The model under review builds one solid part; all positions refer to its coordinate system, in mm. A direction names the side the tool comes from. Coordinates: 2 decimals unless noted, no trailing zeros. Order: outer loops, then holes, each group sorted by start corner. A loop starts at its lowest first (then second) coordinate and runs counter-clockwise, first axis right, second up. Notation, with made-up numbers: (54, -28.75) -> (110, -28.75) arc R4 cw to (110, -21.75) -> close; hole circle Ø2 at (26.5, -18.5). An arc over 180 degrees is marked (long way). Use one line per item in the form item = value. Start each with the question number.
(1) For faces 1 (the flat face through (18.5, -17, -56)), 2 (the flat face through (1, -15.5, -37)), 3 (the flat face through (10, -22, -58)), list the 3-axis set-ups (+Z, -Z, +X, -X, +Y, -Y) from which the entire face can be reached by the end or side of a thin tool; tool diameter is ignored.
(2) Take a section at D-D (z = -17). State the section outline as (x, y) points.
(3) Take a section at C-C (y = 1.5). State the section outline as (x, z) points, then the cut area to 3 significant figures.
(4) Wall thickness on line 1 along Y through (x, z) = (25, 1); line 2 along Y through (x, z) = (-10, 2); line 3 along X through (y, z) = (1, 1): over which ranges is each line inside the solid? List them lowest first.
(5) Insertion check: pin 1 Ø7 at (x, y) = (-10, 8) entering from -Z; pin 2 Ø5 at (x, z) = (-12.5, -7) entering from -Y; pin 3 Ø1.6 at (x, z) = (1.5, -50.5) entering from -Y; pin 4 Ø8 at (x, y) = (-10, -12) entering from -Z. Each pin has a flat end and moves straight along its axis. Give the tip position at first contact, or say it passes through.
(6) Mouldability with a two-part tool opening along X and no side actions: class faces 4 (the flat face through (40, -16, -23)), 5 (the flat face through (1, -34, -50)), 6 (the flat face through (-12, -25, -59)), 7 (the cylindrical face through (20, -17, -60.5)) as +X half, -X half, draft (parallel to the pull), parting line (faces both ways), or undercut.
(7) Take a section at B-B (x = 20). State the section outline as (y, z) points, then the cut area to 3 significant figures.
(8) Take a section at A-A (z = -7). State the section outline as (x, y) points, then the cut area to 3 significant figures.
```python
from build123d import *

# Parameters (mm, degrees)
SZKIC2_W                    = 80
SZKIC2_H                    = 37
SZKIC2_R                    = 3
SZKIC2_R_2                  = 2.5
DODANIE_WYCI_GNI_CIE1_DEPTH = 3
ZAOKR_GLENIE1_R             = 5
SZKIC3_W                    = 80
SZKIC3_H                    = 3
DODANIE_WYCI_GNI_CIE2_DEPTH = 75
WYTNIJ_WYCI_GNI_CIE1_REACH  = 94.704
DODANIE_WYCI_GNI_CIE3_DEPTH = 24
SKORUPA8_START              = -10
SKORUPA8_DEPTH              = 20
SZKIC10_W                   = 20
SZKIC10_H                   = 20
WYTNIJ_WYCI_GNI_CIE5_DEPTH  = 3
SZKIC4_5_R                  = 1.5
WYTNIJ_WYCI_GNI_CIE7_DEPTH  = 3
ZAOKR_GLENIE2_R             = 10
WYTNIJ_WYCI_GNI_CIE8_REACH  = 94.704
SZKIC11_R                   = 2.5


# Read off the part's stored shape, not the designer's step: Skorupa8
with BuildPart() as part:
    # Szkic2 → Dodanie-wyciągnięcie1 (new body)
    with BuildSketch(Plane.XY):
        Rectangle(SZKIC2_W, SZKIC2_H)
        with Locations((-10, -12)):
            Circle(SZKIC2_R, mode=Mode.SUBTRACT)
        with Locations((-25, -8.5)):
            Circle(SZKIC2_R_2, mode=Mode.SUBTRACT)
        with Locations((-25, 1.5)):
            Circle(SZKIC2_R_2, mode=Mode.SUBTRACT)
        with Locations((-25, 11.5)):
            Circle(SZKIC2_R_2, mode=Mode.SUBTRACT)
        with Locations(Location((10, -12, 0), (0, 0, 180))):
            Circle(SZKIC2_R, mode=Mode.SUBTRACT)
        with Locations(Location((25, -8.5, 0), (0, 0, 180))):
            Circle(SZKIC2_R_2, mode=Mode.SUBTRACT)
        with Locations(Location((25, 1.5, 0), (0, 0, 180))):
            Circle(SZKIC2_R_2, mode=Mode.SUBTRACT)
        with Locations(Location((25, 11.5, 0), (0, 0, 180))):
            Circle(SZKIC2_R_2, mode=Mode.SUBTRACT)
        with Locations((-10, 8)):
            Circle(SZKIC2_R, mode=Mode.SUBTRACT)
        with Locations(Location((10, 8, 0), (0, 0, 180))):
            Circle(SZKIC2_R, mode=Mode.SUBTRACT)
    extrude(amount=DODANIE_WYCI_GNI_CIE1_DEPTH)

    # Zaokrąglenie1
    zaokr_glenie1_edges = [part.edges().sort_by_distance(p)[0] for p in [
        (-40, 18.5, 1.5),
        (40, 18.5, 1.5),
    ]]
    fillet(zaokr_glenie1_edges, radius=ZAOKR_GLENIE1_R)

    # Szkic3 → Dodanie-wyciągnięcie2 (add)
    with BuildSketch(Plane(origin=(0, 0, 0), x_dir=(-1, 0, 0), z_dir=(0, 0, -1))):
        with Locations((0, -17)):
            Rectangle(SZKIC3_W, SZKIC3_H)
    extrude(amount=DODANIE_WYCI_GNI_CIE2_DEPTH)

    # Szkic4 → Wytnij-wyciągnięcie1 (cut, up to next)
    with BuildSketch(Plane.XZ.offset(18.5), mode=Mode.PRIVATE) as wytnij_wyci_gni_cie1_sk1:
        with BuildLine():
            Line((-21.5, -65), (-21.5, -70))
            ThreePointArc((-21.5, -70), (-20, -71.5), (-18.5, -70))
            Line((-18.5, -70), (-18.5, -65))
            ThreePointArc((-18.5, -65), (-20, -63.5), (-21.5, -65))
        make_face()
    wytnij_wyci_gni_cie1_tool1 = extrude(wytnij_wyci_gni_cie1_sk1.sketch, amount=-WYTNIJ_WYCI_GNI_CIE1_REACH, mode=Mode.PRIVATE) & part.part
    # Szkic4 → Wytnij-wyciągnięcie1 (cut, up to next)
    with BuildSketch(Plane.XZ.offset(18.5), mode=Mode.PRIVATE) as wytnij_wyci_gni_cie1_sk2:
        with BuildLine():
            ThreePointArc((-18.5, -54), (-20, -52.5), (-21.5, -54))
            Line((-21.5, -54), (-21.5, -59))
            ThreePointArc((-21.5, -59), (-20, -60.5), (-18.5, -59))
            Line((-18.5, -59), (-18.5, -54))
        make_face()
    wytnij_wyci_gni_cie1_tool2 = extrude(wytnij_wyci_gni_cie1_sk2.sketch, amount=-WYTNIJ_WYCI_GNI_CIE1_REACH, mode=Mode.PRIVATE) & part.part
    # Szkic4 → Wytnij-wyciągnięcie1 (cut, up to next)
    with BuildSketch(Plane.XZ.offset(18.5), mode=Mode.PRIVATE) as wytnij_wyci_gni_cie1_sk3:
        with BuildLine():
            ThreePointArc((21.5, -54), (20, -52.5), (18.5, -54))
            Line((18.5, -54), (18.5, -59))
            ThreePointArc((18.5, -59), (20, -60.5), (21.5, -59))
            Line((21.5, -59), (21.5, -54))
        make_face()
    wytnij_wyci_gni_cie1_tool3 = extrude(wytnij_wyci_gni_cie1_sk3.sketch, amount=-WYTNIJ_WYCI_GNI_CIE1_REACH, mode=Mode.PRIVATE) & part.part
    # Szkic4 → Wytnij-wyciągnięcie1 (cut, up to next)
    with BuildSketch(Plane.XZ.offset(18.5), mode=Mode.PRIVATE) as wytnij_wyci_gni_cie1_sk4:
        with BuildLine():
            Line((18.5, -65), (18.5, -70))
            ThreePointArc((18.5, -70), (20, -71.5), (21.5, -70))
            Line((21.5, -70), (21.5, -65))
            ThreePointArc((21.5, -65), (20, -63.5), (18.5, -65))
        make_face()
    wytnij_wyci_gni_cie1_tool4 = extrude(wytnij_wyci_gni_cie1_sk4.sketch, amount=-WYTNIJ_WYCI_GNI_CIE1_REACH, mode=Mode.PRIVATE) & part.part
    add(wytnij_wyci_gni_cie1_tool1.solids().sort_by_distance((-20, -18.5, -67.5))[0], mode=Mode.SUBTRACT)
    add(wytnij_wyci_gni_cie1_tool2.solids().sort_by_distance((-20, -18.5, -56.5))[0], mode=Mode.SUBTRACT)
    add(wytnij_wyci_gni_cie1_tool3.solids().sort_by_distance((20, -18.5, -56.5))[0], mode=Mode.SUBTRACT)
    add(wytnij_wyci_gni_cie1_tool4.solids().sort_by_distance((20, -18.5, -67.5))[0], mode=Mode.SUBTRACT)

    # Szkic8 → Dodanie-wyciągnięcie3 (add)
    with BuildSketch(Plane(origin=(12, 0, 0), x_dir=(0, 0, -1), z_dir=(1, 0, 0))):
        with BuildLine():
            Line((50, -18.5), (50, -35.5))
            ThreePointArc((50, -35.5), (64.90911692, -31.106988593), (74, -18.5))
            Line((74, -18.5), (50, -18.5))
        make_face()
    extrude(amount=-DODANIE_WYCI_GNI_CIE3_DEPTH)

    # Skorupa8 outline → Skorupa8 (cut)
    with BuildSketch(Plane.YZ.offset(SKORUPA8_START)):
        with BuildLine():
            Line((-17.5, -72.209048527), (-17.5, -50))
            Line((-17.5, -50), (-33.497961371, -50))
            ThreePointArc((-33.497961371, -50), (-29.37331804, -63.895346178), (-17.5, -72.209048527))
        make_face()
    extrude(amount=SKORUPA8_DEPTH, mode=Mode.SUBTRACT)

    # Szkic10 → Wytnij-wyciągnięcie5 (cut)
    with BuildSketch(Plane(origin=(0, -15.5, 0), x_dir=(1, 0, 0), z_dir=(0, 1, 0))):
        with Locations((0, 62)):
            Rectangle(SZKIC10_W, SZKIC10_H)
    extrude(amount=-WYTNIJ_WYCI_GNI_CIE5_DEPTH, mode=Mode.SUBTRACT)

    # Szkic4<5> → Wytnij-wyciągnięcie7 (cut)
    with BuildSketch(Plane.XZ.offset(18.5)):
        with Locations(Location((-5.5, -7, 0), (0, 0, 270))):
            Circle(SZKIC4_5_R)
    extrude(amount=-WYTNIJ_WYCI_GNI_CIE7_DEPTH, mode=Mode.SUBTRACT)

    # Zaokrąglenie2
    zaokr_glenie2_edges = [part.edges().sort_by_distance(p)[0] for p in [
        (40, -17, -75),
        (-40, -17, -75),
    ]]
    fillet(zaokr_glenie2_edges, radius=ZAOKR_GLENIE2_R)

    # Szkic11 → Wytnij-wyciągnięcie8 (cut, up to next)
    with BuildSketch(Plane.XZ.offset(18.5), mode=Mode.PRIVATE) as wytnij_wyci_gni_cie8_sk1:
        with Locations(Location((-25, -7, 0), (0, 0, 270))):
            Circle(SZKIC11_R)
    wytnij_wyci_gni_cie8_tool1 = extrude(wytnij_wyci_gni_cie8_sk1.sketch, amount=-WYTNIJ_WYCI_GNI_CIE8_REACH, mode=Mode.PRIVATE) & part.part
    # Szkic11 → Wytnij-wyciągnięcie8 (cut, up to next)
    with BuildSketch(Plane.XZ.offset(18.5), mode=Mode.PRIVATE) as wytnij_wyci_gni_cie8_sk2:
        with Locations(Location((-25, -17, 0), (0, 0, 270))):
            Circle(SZKIC11_R)
    wytnij_wyci_gni_cie8_tool2 = extrude(wytnij_wyci_gni_cie8_sk2.sketch, amount=-WYTNIJ_WYCI_GNI_CIE8_REACH, mode=Mode.PRIVATE) & part.part
    # Szkic11 → Wytnij-wyciągnięcie8 (cut, up to next)
    with BuildSketch(Plane.XZ.offset(18.5), mode=Mode.PRIVATE) as wytnij_wyci_gni_cie8_sk3:
        with Locations(Location((-25, -27, 0), (0, 0, 270))):
            Circle(SZKIC11_R)
    wytnij_wyci_gni_cie8_tool3 = extrude(wytnij_wyci_gni_cie8_sk3.sketch, amount=-WYTNIJ_WYCI_GNI_CIE8_REACH, mode=Mode.PRIVATE) & part.part
    # Szkic11 → Wytnij-wyciągnięcie8 (cut, up to next)
    with BuildSketch(Plane.XZ.offset(18.5), mode=Mode.PRIVATE) as wytnij_wyci_gni_cie8_sk4:
        with Locations(Location((-25, -37, 0), (0, 0, 270))):
            Circle(SZKIC11_R)
    wytnij_wyci_gni_cie8_tool4 = extrude(wytnij_wyci_gni_cie8_sk4.sketch, amount=-WYTNIJ_WYCI_GNI_CIE8_REACH, mode=Mode.PRIVATE) & part.part
    add(wytnij_wyci_gni_cie8_tool1.solids().sort_by_distance((-25, -18.5, -7))[0], mode=Mode.SUBTRACT)
    add(wytnij_wyci_gni_cie8_tool2.solids().sort_by_distance((-25, -18.5, -17))[0], mode=Mode.SUBTRACT)
    add(wytnij_wyci_gni_cie8_tool3.solids().sort_by_distance((-25, -18.5, -27))[0], mode=Mode.SUBTRACT)
    add(wytnij_wyci_gni_cie8_tool4.solids().sort_by_distance((-25, -18.5, -37))[0], mode=Mode.SUBTRACT)


solid = part.part
```
Findings:
q1.face_1 = +Y, -Y
q1.face_2 = -Z, +X, -X, +Y
q1.face_3 = none
q2.outline = (-40, -18.5) -> (-27.5, -18.5) -> (-27.5, -15.5) -> (-40, -15.5) -> close; (-22.5, -18.5) -> (40, -18.5) -> (40, -15.5) -> (-22.5, -15.5) -> close
q3.outline = (-40, 0) -> (-27.5, 0) -> (-27.5, 3) -> (-40, 3) -> close; (-22.5, 0) -> (22.5, 0) -> (22.5, 3) -> (-22.5, 3) -> close; (27.5, 0) -> (40, 0) -> (40, 3) -> (27.5, 3) -> close
q3.area = 210 mm²
q4.line_1 = -18.5 to -11, -6 to -1, 4 to 9, 14 to 18.5
q4.line_2 = -18.5 to -15, -9 to 5, 11 to 18.5
q4.line_3 = -40 to -27.45, -22.55 to 22.55, 27.45 to 40
q5.pin_1 = 0
q5.pin_2 = -18.5
q5.pin_3 = -35.52
q5.pin_4 = -75
q6.face_4 = +X half
q6.face_5 = draft
q6.face_6 = -X half
q6.face_7 = undercut
q7.outline = (-18.5, -75) -> (-15.5, -75) -> (-15.5, -71.5) -> (-18.5, -71.5) -> close; (-18.5, -63.5) -> (-15.5, -63.5) -> (-15.5, -60.5) -> (-18.5, -60.5) -> close; (-18.5, -52.5) -> (-15.5, -52.5) -> (-15.5, 0) -> (18.5, 0) -> (18.5, 3) -> (-18.5, 3) -> close
q7.area = 288 mm²
q8.outline = (-40, -18.5) -> (-27.5, -18.5) -> (-27.5, -15.5) -> (-40, -15.5) -> close; (-22.5, -18.5) -> (-7, -18.5) -> (-7, -15.5) -> (-22.5, -15.5) -> close; (-4, -18.5) -> (40, -18.5) -> (40, -15.5) -> (-4, -15.5) -> close
q8.area = 216 mm²
